Here's how the part is built. I have some questions about the finished solid (model axes, mm). A direction names the side the tool comes from. Give positions to 0.01 mm unless a question says otherwise; leave off trailing zeros. Order: outer loops, then holes, each group sorted by start corner. A loop starts at its lowest first (then second) coordinate and runs counter-clockwise, first axis right, second up. Notation, with made-up numbers: M -15.75,82.5 L 7.25,82.5 A21 cw 7.25,104.5 Z; hole C -28.5,70 d3. An arc over 180 degrees is marked long. Use one line per item in the form item = value.
from build123d import *

# Parameters (mm, degrees)
F0_W     = 50
F0_H     = 40
F1_DEPTH = 6
F2_R     = 2.9
F3_DEPTH = 3.5
F4_R     = 1.6
F5_DEPTH = 25
F6_R     = 1.6
F7_DEPTH = 25
F9_DEPTH = 3.5


with BuildPart() as f1:
    # F0 (on Top) → F1 (new body)
    with BuildSketch(Plane.XY):
        Rectangle(F0_W, F0_H)
    extrude(amount=F1_DEPTH)

    # F2 (on face) → F3 (cut)
    with BuildSketch(Plane.XY.offset(6)):
        with Locations((-9.5, 14)):
            Circle(F2_R)
        with Locations((-9.5, -14)):
            Circle(F2_R)
        with Locations((9.5, 14)):
            Circle(F2_R)
        with Locations((9.5, -14)):
            Circle(F2_R)
    extrude(amount=-F3_DEPTH, mode=Mode.SUBTRACT)

    # F4 (on face) → F5 (cut)
    with BuildSketch(Plane.XY.offset(2.5)):
        with Locations((-9.5, 14)):
            Circle(F4_R)
        with Locations((-9.5, -14)):
            Circle(F4_R)
        with Locations((9.5, 14)):
            Circle(F4_R)
        with Locations((9.5, -14)):
            Circle(F4_R)
    extrude(amount=-F5_DEPTH, mode=Mode.SUBTRACT)

    # F6 (on face) → F7 (cut)
    with BuildSketch(Plane.XY.offset(6)):
        with Locations((-15, 0)):
            Circle(F6_R)
        with Locations((-15, 8)):
            Circle(F6_R)
        with Locations((-15, -8)):
            Circle(F6_R)
        with Locations((15, 0)):
            Circle(F6_R)
        with Locations((15, 8)):
            Circle(F6_R)
        with Locations((15, -8)):
            Circle(F6_R)
        with Locations((-15, -16)):
            Circle(F6_R)
        with Locations((15, 16)):
            Circle(F6_R)
        with Locations((-15, 16)):
            Circle(F6_R)
        with Locations((15, -16)):
            Circle(F6_R)
    extrude(amount=-F7_DEPTH, mode=Mode.SUBTRACT)

    # F8 (on face) → F9 (cut)
    with BuildSketch(Plane(origin=(0, 0, 0), x_dir=(1, 0, 0), z_dir=(0, 0, -1))):
        Polygon((-12.1, -1.674316), (-12.1, 1.674316), (-15, 3.348632), (-17.9, 1.674316), (-17.9, -1.674316), (-15, -3.348632), align=None)
        Polygon((-11.686842, 8.486128), (-13.76442, 11.112343), (-17.077578, 10.626215), (-18.313158, 7.513872), (-16.23558, 4.887657), (-12.922422, 5.373785), align=None)
        Polygon((-11.701039, -7.425379), (-13.848156, -4.855705), (-17.147117, -5.430327), (-18.298961, -8.574621), (-16.151844, -11.144295), (-12.852883, -10.569673), align=None)
        Polygon((17.9, -1.674316), (17.9, 1.674316), (15, 3.348632), (12.1, 1.674316), (12.1, -1.674316), (15, -3.348632), align=None)
        Polygon((18.313158, 8.486128), (16.23558, 11.112343), (12.922422, 10.626215), (11.686842, 7.513872), (13.76442, 4.887657), (17.077578, 5.373785), align=None)
        Polygon((18.298961, -7.425379), (16.151844, -4.855705), (12.852883, -5.430327), (11.701039, -8.574621), (13.848156, -11.144295), (17.147117, -10.569673), align=None)
        Polygon((-12.03478, 17.555894), (-14.864834, 19.345902), (-17.830053, 17.790009), (-17.96522, 14.444106), (-15.135166, 12.654098), (-12.169947, 14.209991), align=None)
        Polygon((-17.9, -14.325684), (-17.9, -17.674316), (-15, -19.348632), (-12.1, -17.674316), (-12.1, -14.325684), (-15, -12.651368), align=None)
        Polygon((18.144295, 14.848156), (17.569673, 18.147117), (14.425379, 19.298961), (11.855705, 17.151844), (12.430327, 13.852883), (15.574621, 12.701039), align=None)
        Polygon((18.144295, -17.151844), (17.569673, -13.852883), (14.425379, -12.701039), (11.855705, -14.848156), (12.430327, -18.147117), (15.574621, -19.298961), align=None)
    extrude(amount=-F9_DEPTH, mode=Mode.SUBTRACT)


solid = f1.part
Q1. I want a section at A-A on x = 9.5. Write out the boundary of the cut face in (y, z).
Found:
outline = M -20,0 L -15.6,0 L -15.6,2.5 L -16.9,2.5 L -16.9,6 L -20,6 Z; M -12.4,0 L 12.4,0 L 12.4,2.5 L 11.1,2.5 L 11.1,6 L -11.1,6 L -11.1,2.5 L -12.4,2.5 Z; M 15.6,0 L 20,0 L 20,6 L 16.9,6 L 16.9,2.5 L 15.6,2.5 Z
Q2. On a 3-axis mill with a long thin cutter (end or side, diameter ignored), from which of +Z, -Z, +X, -X, +Y, -Y can I reach the whole of each face in a straight line? I mean faces 1 (the face through (-8, 13, 2.5)), 2 (the face through (8.32, 15.08, 1.27)), 3 (the face through (-14.53, 10.86, 1.73)). Say none if no direction works.
Found:
face_1 = +Z
face_2 = +Z, -Z
face_3 = -Z
Q3. I need wall thicknesses on L1, parallel to X at y = 0, z = 2.65; L2, parallel to Y at x = -9.5, z = 4.6; L3, parallel to X at y = -14, z = 4.55. Which ranges of each line are inside material? Lowest first, please.
Found:
L1 = -25 to -17.9, -12.1 to 12.1, 17.9 to 25
L2 = -20 to -16.9, -11.1 to 11.1, 16.9 to 20
L3 = -25 to -12.4, -6.6 to 6.6, 12.4 to 25
Q4. I want a section at B-B on z = 5.3. State how many separate pieces and enclosed holes the cut face has, then the cut area to 3 significant figures.
Found:
separate_pieces = 1
enclosed_holes = 14
area = 1,810 mm²
Q5. I'm going to push flat-ended pins straight in: pin 1 Ø3 at (x, y) = (-16, -8) entering from -Z; pin 2 Ø6.5 at (x, y) = (-10, 15) entering from +Z; pin 3 Ø3 at (x, y) = (9, -14.5) entering from +Z. Where does each tip first touch, or does it pass through?
Found:
pin_1 = 3.5
pin_2 = 6
pin_3 = 2.5
